Build history of the part. All positions in model axes, mm. Face numbers are marked on the shaded views. A direction names the side the tool comes from. Give positions to 0.01 mm unless a question says otherwise; leave off trailing zeros. Order: outer loops, then holes, each group sorted by start corner. A loop starts at its lowest first (then second) coordinate and runs counter-clockwise, first axis right, second up. Notation, with made-up numbers: (51, -12.5) - (75, -12.5) arc R22 ccw to (75, 6.5) - close; hole circle Ø5 at (87, 65). An arc over 180 degrees is marked (long way). Answer in a Markdown table with one row per item.
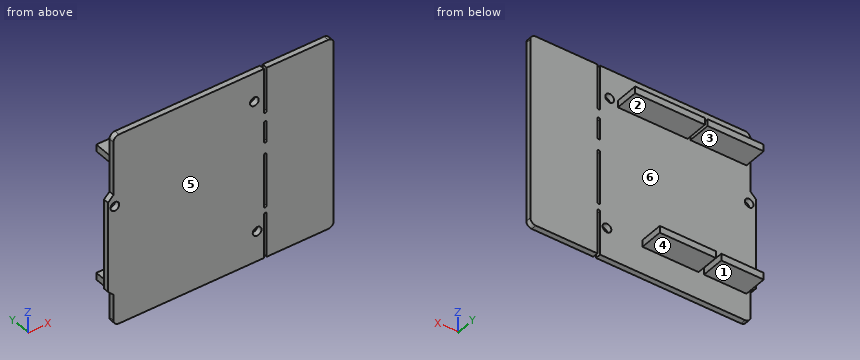
```python
from build123d import *

# Parameters (mm, degrees)
SZKIC2_R                    = 1.6
DODANIE_WYCI_GNI_CIE1_DEPTH = 2
SZKIC3_W                    = 15.5
SZKIC3_H                    = 2.5
SZKIC3_W_2                  = 20.5
SZKIC3_W_3                  = 25.5
DODANIE_WYCI_GNI_CIE2_DEPTH = 8.5


with BuildPart() as part:
    # Szkic2 → Dodanie-wyciągnięcie1 (new body)
    with BuildSketch(Plane(origin=(0, 0, 0), x_dir=(1, 0, 0), z_dir=(0, 1, 0))):
        with BuildLine():
            Line((-43.319305218, 25.801941522), (-43.319305218, -7.198058478))
            Line((-43.319305218, -7.198058478), (-41.319305218, -9.198058478))
            Line((-41.319305218, -9.198058478), (-41.319305218, -28.698058478))
            ThreePointArc((-41.319305218, -28.698058478), (-40.73351878, -30.11227204), (-39.319305218, -30.698058478))
            Line((-39.319305218, -30.698058478), (13.680694782, -30.698058478))
            Line((13.680694782, -30.698058478), (13.680694782, -14.698058478))
            ThreePointArc((13.680694782, -14.698058478), (14.180694782, -14.198058478), (14.680694782, -14.698058478))
            Line((14.680694782, -14.698058478), (14.680694782, -30.698058478))
            Line((14.680694782, -30.698058478), (37.180694782, -30.698058478))
            ThreePointArc((37.180694782, -30.698058478), (38.594908344, -30.11227204), (39.180694782, -28.698058478))
            Line((39.180694782, -28.698058478), (39.180694782, 37.301941522))
            ThreePointArc((39.180694782, 37.301941522), (38.594908344, 38.716155084), (37.180694782, 39.301941522))
            Line((37.180694782, 39.301941522), (14.680694782, 39.301941522))
            Line((14.680694782, 39.301941522), (14.680694782, 23.301941522))
            ThreePointArc((14.680694782, 23.301941522), (14.180694782, 22.801941522), (13.680694782, 23.301941522))
            Line((13.680694782, 23.301941522), (13.680694782, 39.301941522))
            Line((13.680694782, 39.301941522), (-39.319305218, 39.301941522))
            ThreePointArc((-39.319305218, 39.301941522), (-40.73351878, 38.716155084), (-41.319305218, 37.301941522))
            Line((-41.319305218, 37.301941522), (-41.319305218, 27.801941522))
            Line((-41.319305218, 27.801941522), (-43.319305218, 25.801941522))
        make_face()
        with Locations(Location((-40.819305218, -4.698058478, 0), (0, 0, 270))):
            Circle(SZKIC2_R, mode=Mode.SUBTRACT)
        with Locations(Location((10.180694782, -20.198058478, 0), (0, 0, 270))):
            Circle(SZKIC2_R, mode=Mode.SUBTRACT)
        with BuildLine():
            ThreePointArc((13.680694782, -3.698058478), (14.180694782, -3.198058478), (14.680694782, -3.698058478))
            Line((14.680694782, -3.698058478), (14.680694782, -10.698058478))
            ThreePointArc((14.680694782, -10.698058478), (14.180694782, -11.198058478), (13.680694782, -10.698058478))
            Line((13.680694782, -10.698058478), (13.680694782, -3.698058478))
        make_face(mode=Mode.SUBTRACT)
        with BuildLine():
            ThreePointArc((13.680694782, 20.301941522), (14.180694782, 20.801941522), (14.680694782, 20.301941522))
            Line((14.680694782, 20.301941522), (14.680694782, 1.301941522))
            ThreePointArc((14.680694782, 1.301941522), (14.180694782, 0.801941522), (13.680694782, 1.301941522))
            Line((13.680694782, 1.301941522), (13.680694782, 20.301941522))
        make_face(mode=Mode.SUBTRACT)
        with Locations(Location((11.180694782, 28.301941522, 0), (0, 0, 270))):
            Circle(SZKIC2_R, mode=Mode.SUBTRACT)
    extrude(amount=DODANIE_WYCI_GNI_CIE1_DEPTH)

    # Szkic3 → Dodanie-wyciągnięcie2 (add)
    with BuildSketch(Plane(origin=(0, 2, 0), x_dir=(1, 0, 0), z_dir=(0, 1, 0))):
        with Locations((-32.069305218, 28.051941522)):
            Rectangle(SZKIC3_W, SZKIC3_H)
        with Locations((-12.069305218, 28.051941522)):
            Rectangle(SZKIC3_W_2, SZKIC3_H)
        with Locations((-29.569305218, -19.448058478)):
            Rectangle(SZKIC3_W_2, SZKIC3_H)
        with Locations((-5.569305218, -19.448058478)):
            Rectangle(SZKIC3_W_3, SZKIC3_H)
    extrude(amount=DODANIE_WYCI_GNI_CIE2_DEPTH)


solid = part.part
```
1. Cut at D-D on x = 3.5. Write the cut outline in (y, z).
Check result:
| item | result |
|---|---|
| outline | (0, -39.3) - (2, -39.3) - (2, 18.2) - (10.5, 18.2) - (10.5, 20.7) - (2, 20.7) - (2, 30.7) - (0, 30.7) - close |
2. Cut at B-B on y = 6.75. Write the cut outline in (x, z), and give its area (3 significant figures).
Check result:
| item | result |
|---|---|
| outline | (-39.82, -29.3) - (-24.32, -29.3) - (-24.32, -26.8) - (-39.82, -26.8) - close; (-39.82, 18.2) - (-19.32, 18.2) - (-19.32, 20.7) - (-39.82, 20.7) - close; (-22.32, -29.3) - (-1.82, -29.3) - (-1.82, -26.8) - (-22.32, -26.8) - close; (-18.32, 18.2) - (7.18, 18.2) - (7.18, 20.7) - (-18.32, 20.7) - close |
| area | 205 mm² |
3. Cut at A-A on z = 25. Write the cut outline in (x, y), and give its area (3 significant figures).
Check result:
| item | result |
|---|---|
| outline | (-41.32, 0) - (13.68, 0) - (13.68, 2) - (-41.32, 2) - close; (14.68, 0) - (39.18, 0) - (39.18, 2) - (14.68, 2) - close |
| area | 159 mm² |
4. Probe line 1 (Z direction, x = -30, y = 4.5); line 2 (X direction, y = 0.5, z = 10); line 3 (Z direction, x = 11, y = 1). List the from-to ranges inside material, lowest first.
Check result:
| item | result |
|---|---|
| line 1 | z = -29.3 to -26.8, 18.2 to 20.7 |
| line 2 | x = -41.32 to 13.68, 14.68 to 39.18 |
| line 3 | z = -39.3 to -29.89, -26.71 to 18.82, 21.57 to 30.7 |
5. Two-plate mould, pull along Z, no slides. Class the marked faces 3, 4, 5 and 6: +Z half, -Z half, draft (parallel to the pull), parting line (faces both ways), or undercut.
Check result:
| item | result |
|---|---|
| face 3 | undercut |
| face 4 | -Z half |
| face 5 | draft |
| face 6 | undercut |
6. Cut at C-C on x = -29. Write the cut outline in (y, z).
Check result:
| item | result |
|---|---|
| outline | (0, -39.3) - (2, -39.3) - (2, -29.3) - (10.5, -29.3) - (10.5, -26.8) - (2, -26.8) - (2, 18.2) - (10.5, 18.2) - (10.5, 20.7) - (2, 20.7) - (2, 30.7) - (0, 30.7) - close |
7. Which spindle directions (+Z, -Z, +X, -X, +Y, -Y) get a long thin tool onto all of the face, cutting with end or side? Do the marked faces 1 and 2. Say none if no direction does.
Check result:
| item | result |
|---|---|
| face 1 | -Z, +X, -X, +Y |
| face 2 | +X, -X, +Y |
8. Drop flat-ended pins along their axis: P1, Ø3, axis at x = -32, z = -25, coming from the +Y side; P2, Ø4, axis at x = -31, y = 7.5, coming from the -Z side; P3, Ø2, axis at y = 6, z = 20, coming from the -X side. Give the stop position or say it passes through.
Check result:
| item | result |
|---|---|
| P1 | stops at y = 2 |
| P2 | stops at z = -29.3 |
| P3 | stops at x = -39.82 |
